```python
from build123d import *

# Parameters (mm, degrees)
F1_DEPTH = 25.4
F3_DEPTH = 9.878778
F5_DEPTH = 17.904465
F7_DEPTH = 17.904465
F8_R     = 6.35
F9_DEPTH = 9.878778


with BuildPart() as f1:
    # F0 (on Front) → F1 (new body)
    with BuildSketch(Plane.XZ):
        Polygon((-72.174763, 57.95379), (-72.174763, 13.50379), (-9.821297, 13.50379), (-9.821297, 23.381569), (-54.271297, 23.381569), (-54.271297, 57.95379), align=None)
    extrude(amount=F1_DEPTH)

    # F2 (on face) → F3 (cut, through all)
    with BuildSketch(Plane.XY.offset(23.381569)):
        with BuildLine():
            Line((-9.821297, -12.7), (-9.821297, 0))
            Line((-9.821297, 0), (-22.521297, 0))
            ThreePointArc((-22.521297, 0), (-13.541041, -3.719744), (-9.821297, -12.7))
        make_face()
        with BuildLine():
            Line((-9.821297, -25.4), (-9.821297, -12.7))
            ThreePointArc((-9.821297, -12.7), (-13.541041, -21.680256), (-22.521297, -25.4))
            Line((-22.521297, -25.4), (-9.821297, -25.4))
        make_face()
    extrude(amount=-F3_DEPTH, mode=Mode.SUBTRACT)

    # F4 (on face) → F5 (cut, through all)
    with BuildSketch(Plane.YZ.offset(-54.271297)):
        with BuildLine():
            Line((-12.7, 57.95379), (-25.4, 57.95379))
            Line((-25.4, 57.95379), (-25.4, 45.25379))
            ThreePointArc((-25.4, 45.25379), (-21.680256, 54.234047), (-12.7, 57.95379))
        make_face()
        with BuildLine():
            Line((0, 57.95379), (-12.7, 57.95379))
            ThreePointArc((-12.7, 57.95379), (-3.719744, 54.234047), (0, 45.25379))
            Line((0, 45.25379), (0, 57.95379))
        make_face()
    extrude(amount=-F5_DEPTH, mode=Mode.SUBTRACT)

    # F6 (on face) → F7 (cut, through all)
    with BuildSketch(Plane.YZ.offset(-54.271297)):
        with BuildLine():
            ThreePointArc((-19.042094, 45.570553), (-12.625386, 51.603352), (-6.352213, 45.421435))
            Line((-6.352213, 45.421435), (-6.642582, 56.416124))
            ThreePointArc((-6.642582, 56.416124), (-12.863096, 57.952743), (-19.042094, 56.256874))
            Line((-19.042094, 56.256874), (-19.042094, 45.570553))
        make_face()
        with BuildLine():
            ThreePointArc((-19.042094, 44.937028), (-12.541569, 38.905767), (-6.35, 45.25379))
            ThreePointArc((-6.35, 45.25379), (-6.350553, 45.33762), (-6.352213, 45.421435))
            ThreePointArc((-6.352213, 45.421435), (-12.625386, 51.603352), (-19.042094, 45.570553))
            Line((-19.042094, 45.570553), (-19.042094, 44.937028))
        make_face()
    extrude(amount=-F7_DEPTH, mode=Mode.SUBTRACT)

    # F8 (on face) → F9 (cut, through all)
    with BuildSketch(Plane.XY.offset(23.381569)):
        with Locations((-41.571297, -12.7)):
            Circle(F8_R)
        with Locations((-22.521297, -12.7)):
            Circle(F8_R)
    extrude(amount=-F9_DEPTH, mode=Mode.SUBTRACT)


solid = f1.part
```
Check sheet for the modelled part. Datum: model origin and axes. Units: mm. A direction names the side the tool comes from. Round coordinates to 2 decimals unless told otherwise and drop trailing zeros. Write each loop counter-clockwise with the first axis right and the second up, starting at its lowest first coordinate (ties: lowest second). Pieces come first, ordered by that corner, then holes. Notation, with made-up numbers: (43.25, -2.5) -> (69.25, -2.5) arc R15 cw to (69.25, 10.5) -> close; hole circle Ø11 at (-39.5, 61.5). An arc over 180 degrees is marked (long way). One line per question, with ' | ' between items. Start each with the question number.
1. Sectioned sample at B-B, the plane y = -14. Record the cut outline in (x, z).
2. Scan lines: line 1 along Z through (x, y) = (-14, -19.75); line 2 along X through (y, z) = (-8.5, 37.5); line 3 along Y through (x, z) = (-40.5, 20). Record each from-to range of solid material in increasing order. Write a range as from..to.
3. Set-up check for faces 4 (the face through (-63, -19.042, 51)), 5 (the face through (-32, -13, 23.382)), 6 (the face through (-23.9, -18.9, 18.5)): record each of +Z, -Z, +X, -X, +Y, -Y from which the full face is reachable in a straight line by a thin tool's end or side.
4. Sectioned sample at A-A, the plane x = -44. Record the cut outline in (y, z), then the cut area to 3 significant figures.
5. Depth check by flat-ended pin: pin 1 (1.5 mm diameter, centred on x = -60.5, z = 52, fed in from +Y); pin 2 (10 mm diameter, centred on y = -5, z = 36, fed in from +X); pin 3 (2 mm diameter, centred on x = -24.5, y = -21, fed in from +Z). Enter the tip coordinate at first touch or a pass-through.
6. Sectioned sample at C-C, the plane z = 41. Record the cut outline in (x, y).
7. Sectioned sample at D-D, the plane x = -61. Record the cut outline in (y, z), then the cut area to 3 significant figures.
8. Release check for a two-part mould opening along Y. For faces 1 (the face through (-53, 0, 23)), 2 (the face through (-54.271, -13, 36)), 3 (the face through (-47.915, -12.421, 18.512)) record: +Y half, -Y half, draft (parallel to the pull), parting line (faces both ways), or undercut.
Taken from the geometry:
1) outline: (-72.17, 13.5) -> (-47.79, 13.5) -> (-47.79, 23.38) -> (-54.27, 23.38) -> (-54.27, 39.04) -> (-72.17, 39.04) -> close; (-35.36, 13.5) -> (-28.74, 13.5) -> (-28.74, 23.38) -> (-35.36, 23.38) -> close; (-16.31, 13.5) -> (-9.89, 13.5) -> (-9.89, 23.38) -> (-16.31, 23.38) -> close
2) line 1: z = 13.5..23.38 | line 2: x = -72.17..-54.27 | line 3: y = -25.4..-18.96, -6.44..0
3) face 4: +Z, +X, -X | face 5: +Z, +X, +Y, -Y | face 6: +Z, -Z
4) outline: (-25.4, 13.5) -> (-18.57, 13.5) -> (-18.57, 23.38) -> (-25.4, 23.38) -> close; (-6.83, 13.5) -> (0, 13.5) -> (0, 23.38) -> (-6.83, 23.38) -> close | area: 135 mm^2
5) pin 1: stops at y = -1.5 | pin 2: stops at x = -54.27 | pin 3: stops at z = 23.38
6) outline: (-72.17, -25.4) -> (-54.27, -25.4) -> (-54.27, -17.41) -> (-72.17, -17.41) -> close; (-72.17, -7.99) -> (-54.27, -7.99) -> (-54.27, 0) -> (-72.17, 0) -> close
7) outline: (-25.4, 13.5) -> (0, 13.5) -> (0, 45.25) arc R12.7 ccw to (-6.64, 56.42) -> (-6.35, 45.42) arc R6.35 cw to (-6.35, 45.25) arc R6.35 cw to (-19.04, 44.94) -> (-19.04, 56.26) arc R12.7 ccw to (-25.4, 45.25) -> close | area: 844 mm^2
8) face 1: +Y half | face 2: draft | face 3: undercut
